from build123d import *

# Parameters (mm, degrees)
SKETCH1_W           = 45
SKETCH1_H           = 45
BOSS_EXTRUDE1_DEPTH = 25
SKETCH2_W           = 20
SKETCH2_H           = 20
CUT_EXTRUDE1_DEPTH  = 187.975674979
SKETCH3_W           = 25
SKETCH3_H           = 25
SKETCH3_W_2         = 23
SKETCH3_H_2         = 23
CUT_EXTRUDE2_DEPTH  = 20
SKETCH4_W           = 25
SKETCH4_H           = 25
SKETCH4_W_2         = 23
SKETCH4_H_2         = 23
CUT_EXTRUDE3_DEPTH  = 20
SKETCH7_W           = 19
SKETCH7_H           = 19
CUT_EXTRUDE7_DEPTH  = 42
SKETCH8_W           = 19
SKETCH8_H           = 19
CUT_EXTRUDE8_DEPTH  = 42


with BuildPart() as part:
    # Sketch1 → Boss-Extrude1 (new body)
    with BuildSketch(Plane.XY):
        with Locations((-22.649542037, -157.212052706)):
            Rectangle(SKETCH1_W, SKETCH1_H)
    extrude(amount=BOSS_EXTRUDE1_DEPTH)

    # Sketch2 → Cut-Extrude1 (cut, through all)
    with BuildSketch(Plane.XY.offset(25)):
        with Locations((-10.149542037, -169.712052706)):
            Rectangle(SKETCH2_W, SKETCH2_H)
    extrude(amount=-CUT_EXTRUDE1_DEPTH, mode=Mode.SUBTRACT)

    # Sketch3 → Cut-Extrude2 (cut)
    with BuildSketch(Plane(origin=(-0.149542037, 0, 0), x_dir=(0, 0, -1), z_dir=(1, 0, 0))):
        with Locations((-12.5, -147.212052706)):
            Rectangle(SKETCH3_W, SKETCH3_H)
        with Locations((-12.5, -147.212052706)):
            Rectangle(SKETCH3_W_2, SKETCH3_H_2, mode=Mode.SUBTRACT)
    extrude(amount=-CUT_EXTRUDE2_DEPTH, mode=Mode.SUBTRACT)

    # Sketch4 → Cut-Extrude3 (cut)
    with BuildSketch(Plane.XZ.offset(179.712052706)):
        with Locations((-32.649542037, 12.5)):
            Rectangle(SKETCH4_W, SKETCH4_H)
        with Locations((-32.649542037, 12.5)):
            Rectangle(SKETCH4_W_2, SKETCH4_H_2, mode=Mode.SUBTRACT)
    extrude(amount=-CUT_EXTRUDE3_DEPTH, mode=Mode.SUBTRACT)

    # Sketch7 → Cut-Extrude7 (cut)
    with BuildSketch(Plane(origin=(-0.149542037, 0, 0), x_dir=(0, 0, -1), z_dir=(1, 0, 0))):
        with Locations((-12.5, -147.212052706)):
            Rectangle(SKETCH7_W, SKETCH7_H)
    extrude(amount=-CUT_EXTRUDE7_DEPTH, mode=Mode.SUBTRACT)

    # Sketch8 → Cut-Extrude8 (cut)
    with BuildSketch(Plane.XZ.offset(179.712052706)):
        with Locations((-32.649542037, 12.5)):
            Rectangle(SKETCH8_W, SKETCH8_H)
    extrude(amount=-CUT_EXTRUDE8_DEPTH, mode=Mode.SUBTRACT)


solid = part.part
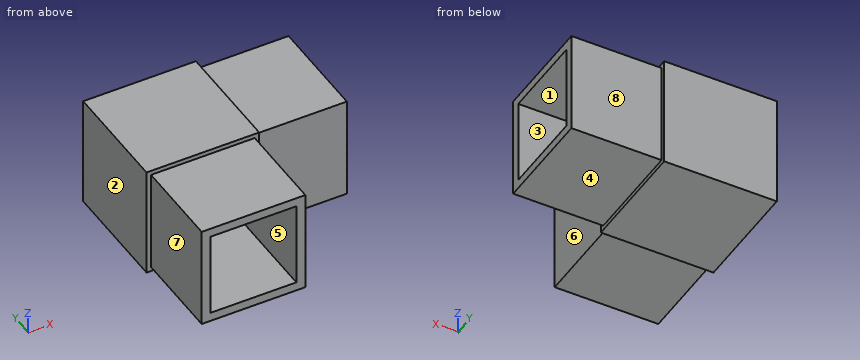
Model file for the job. Use its own axes, mm. Face numbers are marked on the shaded views. A direction names the side the tool comes from. Give positions to 0.01 mm unless a question says otherwise; leave off trailing zeros. Order: outer loops, then holes, each group sorted by start corner. A loop starts at its lowest first (then second) coordinate and runs counter-clockwise, first axis right, second up. Notation, with made-up numbers: (-12.75, 63) - (41.25, 63) arc R24 ccw to (41.25, 88) - close; hole circle Ø3 at (-27, -21.5). An arc over 180 degrees is marked (long way). One line per item, written item: value.
Item 1: Wall check: line 1 (Y direction, x = -11, z = 21); line 2 (X direction, y = -162.5, z = 19); line 3 (Z direction, x = -34, y = -161). Give the ranges that are in metal, low to high.
Response values:
line 1: -158.71 to -156.71, -137.71 to -135.71
line 2: -44.15 to -42.15, -23.15 to -21.15
line 3: 1 to 3, 22 to 24
Item 2: Two-plate mould, pull along X, no slides. Class the marked faces 1, 2 and 3: released by +X, released by -X, zero draft, split by the parting line, or undercut.
Response values:
face 1: undercut
face 2: released by -X
face 3: zero draft
Item 3: Pin check, flat tips, straight feed: pin 1 Ø8 at (x, z) = (-10.5, 22.5) entering from +Y; pin 2 Ø5.5 at (x, z) = (-27, 8.5) entering from -Y; pin 3 Ø9.5 at (y, z) = (-173.5, 10) entering from -X. Stop position of each tip, or through.
Response values:
pin 1: y = -135.71
pin 2: y = -137.71
pin 3: x = -44.15
Item 4: Slice it at D-D (x = -41). List the corners of the cut face in (y, z).
Response values:
outline: (-179.71, 1) - (-159.71, 1) - (-159.71, 0) - (-134.71, 0) - (-134.71, 25) - (-159.71, 25) - (-159.71, 24) - (-179.71, 24) - (-179.71, 22) - (-137.71, 22) - (-137.71, 3) - (-179.71, 3) - close
Item 5: Tool access for the marked faces 4, 5, 6, 7 and 8: list every direction of +Z, -Z, +X, -X, +Y, -Y with a clear straight run to the whole face (end or side of a thin tool).
Response values:
face 4: -Z, +X, +Y, -Y
face 5: -Y
face 6: +Z, -Z, +X, -Y
face 7: +Z, -Z, -X, -Y
face 8: +Z, -Z, +X, +Y
Item 6: Slice it at C-C (y = -140.5). List the corners of the cut face in (x, z), then the cut area to 3 significant figures.
Response values:
outline: (-45.15, 0) - (-20.15, 0) - (-20.15, 1) - (-0.15, 1) - (-0.15, 3) - (-42.15, 3) - (-42.15, 22) - (-0.15, 22) - (-0.15, 24) - (-20.15, 24) - (-20.15, 25) - (-45.15, 25) - close
area: 287 mm2
Item 7: Slice it at A-A (z = 8). List the corners of the cut face in (x, y).
Response values:
outline: (-45.15, -159.71) - (-44.15, -159.71) - (-44.15, -179.71) - (-42.15, -179.71) - (-42.15, -137.71) - (-0.15, -137.71) - (-0.15, -135.71) - (-20.15, -135.71) - (-20.15, -134.71) - (-45.15, -134.71) - close; (-23.15, -179.71) - (-21.15, -179.71) - (-21.15, -159.71) - (-20.15, -159.71) - (-20.15, -158.71) - (-0.15, -158.71) - (-0.15, -156.71) - (-23.15, -156.71) - close
Item 8: Slice it at B-B (x = -17.5). List the corners of the cut face in (y, z), then the cut area to 3 significant figures.
Response values:
outline: (-158.71, 1) - (-135.71, 1) - (-135.71, 24) - (-158.71, 24) - close; hole (-156.71, 3) - (-137.71, 3) - (-137.71, 22) - (-156.71, 22) - close
area: 168 mm2
